Work out the finished part from the listing and answer in its coordinate system (mm). Face numbers are marked on the shaded views. Give positions to 0.01 mm unless a question says otherwise; leave off trailing zeros. Loops run counter-clockwise (first coordinate to the right, second up) from the corner with the lowest first, then second, coordinate; pieces in that order, holes last.
```python
from build123d import *

# Parameters (mm, degrees)
SKETCH_1_W          = 15
SKETCH_1_H          = 15
SKETCH_1_W_2        = 12
SKETCH_1_H_2        = 12
EXTRUDE_1_DEPTH     = 220
SKETCH_2_R          = 2.1
CUT_EXTRUDE_1_DEPTH = 221.638278637
SKETCH_3_R          = 2.1
CUT_EXTRUDE_2_DEPTH = 221.638278637
SKETCH_4_R          = 2.1
CUT_EXTRUDE_3_DEPTH = 221.638278637
SKETCH_5_R          = 2.1
CUT_EXTRUDE_4_DEPTH = 221.638278637
SKETCH_6_R          = 2.1
CUT_EXTRUDE_5_DEPTH = 221.638278637


with BuildPart() as part:
    # ｽｹｯﾁ1 → 押し出し-薄板1 (new body)
    with BuildSketch(Plane(origin=(0, 0, 0), x_dir=(1, 0, 0), z_dir=(0, 1, 0))):
        Rectangle(SKETCH_1_W, SKETCH_1_H)
        Rectangle(SKETCH_1_W_2, SKETCH_1_H_2, mode=Mode.SUBTRACT)
    extrude(amount=EXTRUDE_1_DEPTH)

    # ｽｹｯﾁ2 → ｶｯﾄ - 押し出し1 (cut, through all)
    with BuildSketch(Plane(origin=(7.5, 0, 0), x_dir=(0, 0, -1), z_dir=(1, 0, 0))):
        with Locations((0, 215)):
            Circle(SKETCH_2_R)
    extrude(amount=-CUT_EXTRUDE_1_DEPTH, mode=Mode.SUBTRACT)

    # ｽｹｯﾁ3 → ｶｯﾄ - 押し出し2 (cut, through all)
    with BuildSketch(Plane(origin=(7.5, 0, 0), x_dir=(0, 0, -1), z_dir=(1, 0, 0))):
        with Locations((0, 145)):
            Circle(SKETCH_3_R)
        with Locations((0, 180)):
            Circle(SKETCH_3_R)
    extrude(amount=-CUT_EXTRUDE_2_DEPTH, mode=Mode.SUBTRACT)

    # ｽｹｯﾁ4 → ｶｯﾄ - 押し出し3 (cut, through all)
    with BuildSketch(Plane.XY.offset(7.5)):
        with Locations((0, 205)):
            Circle(SKETCH_4_R)
    extrude(amount=-CUT_EXTRUDE_3_DEPTH, mode=Mode.SUBTRACT)

    # ｽｹｯﾁ5 → ｶｯﾄ - 押し出し4 (cut, through all)
    with BuildSketch(Plane.XY.offset(7.5)):
        with Locations((0, 22.5)):
            Circle(SKETCH_5_R)
        with Locations((0, 7.5)):
            Circle(SKETCH_5_R)
    extrude(amount=-CUT_EXTRUDE_4_DEPTH, mode=Mode.SUBTRACT)

    # ｽｹｯﾁ6 → ｶｯﾄ - 押し出し5 (cut, through all)
    with BuildSketch(Plane(origin=(7.5, 0, 0), x_dir=(0, 0, -1), z_dir=(1, 0, 0))):
        with Locations((0, 80)):
            Circle(SKETCH_6_R)
        with Locations((0, 127.5)):
            Circle(SKETCH_6_R)
    extrude(amount=-CUT_EXTRUDE_5_DEPTH, mode=Mode.SUBTRACT)


solid = part.part
```
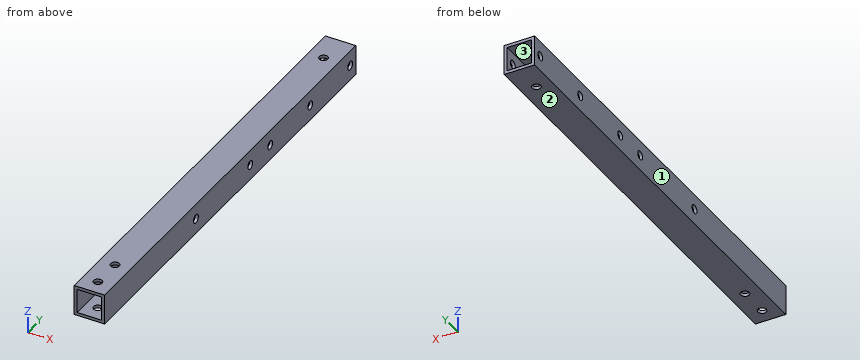
Q1. Consider line 1 along Y through (x, z) = (-7.2, 0); line 2 along Y through (x, z) = (0, 6.7); line 3 along Z through (x, y) = (-4.5, 193). Determine where each line is inside the solid, lowest interval first.
Q2. Determine the mould class of the marked faces 1, 2 and 3 for opening direction X: +X half, -X half, draft (parallel to the pull), parting line (faces both ways), or undercut.
Q3. Section D-D on z = 0 is taken. State how many separate pieces and enclosed holes the cut face has, plus the area to 3 significant figures.
Q4. Section A-A on x = -4 is taken. Give the vertices of the cut face in (y, z).
Q5. Section C-C on y = 113 is taken. Give the vertices of the cut face in (x, z), plus the area to 3 significant figures.
Q6. Section B-B on y = 80 is taken. Give the vertices of the cut face in (x, z).
Q7. Given pin 1 (3.5 mm diameter, centred on y = 215, z = 0, fed in from +X), flat-ended and moving along its own axis, determine where the tip first touches the part or whether it passes through.
Check result:
1. line 1: y = 0 to 77.9, 82.1 to 125.4, 129.6 to 142.9, 147.1 to 177.9, 182.1 to 212.9, 217.1 to 220
1. line 2: y = 0 to 5.4, 9.6 to 20.4, 24.6 to 202.9, 207.1 to 220
1. line 3: z = -7.5 to -6, 6 to 7.5
2. face 1: -X half
2. face 2: draft
2. face 3: undercut
3. separate pieces: 12
3. enclosed holes: 0
3. area: 597 mm2
4. outline: (0, -7.5) - (220, -7.5) - (220, -6) - (0, -6) - close; (0, 6) - (220, 6) - (220, 7.5) - (0, 7.5) - close
5. outline: (-7.5, -7.5) - (7.5, -7.5) - (7.5, 7.5) - (-7.5, 7.5) - close; hole (-6, -6) - (6, -6) - (6, 6) - (-6, 6) - close
5. area: 81.0 mm2
6. outline: (-7.5, -7.5) - (7.5, -7.5) - (7.5, -2.1) - (6, -2.1) - (6, -6) - (-6, -6) - (-6, -2.1) - (-7.5, -2.1) - close; (-7.5, 2.1) - (-6, 2.1) - (-6, 6) - (6, 6) - (6, 2.1) - (7.5, 2.1) - (7.5, 7.5) - (-7.5, 7.5) - close
7. pin 1: passes through
